Build history of the part. All positions in model axes, mm. Face numbers are marked on the shaded views. A direction names the side the tool comes from. Give positions to 0.01 mm unless a question says otherwise; leave off trailing zeros. Loops run counter-clockwise (first coordinate to the right, second up) from the corner with the lowest first, then second, coordinate; pieces in that order, holes last. Notation, with made-up numbers: (-16.75, 66.25) -> (13.25, 66.25) arc R11 ccw to (13.25, 70.25) -> close; hole circle Ø8 at (-10, 66). An arc over 180 degrees is marked (long way). Answer as a JSON object with one key per item and string values. Group by question number.
Q1. Two-plate mould, pull along X, no slides. Class the marked faces 3, 4, 5 and 6: pulls with the +X half, pulls with the -X half, needs draft (parallel to the pull), parting line crosses it, or undercut.
Q2. Wall check: probe 1 along Y at (x, z) = (-20, 0.5); probe 2 along Y at (x, z) = (21.5, 0.85). Give the ranges that are in metal, low to high. Write a range as from..to.
Q3. Tool access for the marked faces 1 and 2: list every direction of +Z, -Z, +X, -X, +Y, -Y with a clear straight run to the whole face (end or side of a thin tool).
Q4. Band-saw the part on B-B, the plane x = 26. Write the cut outline in (y, z), plus the area to 3 significant figures.
Q5. Band-saw the part on A-A, the plane y = 1.4. Count the separate pieces of the cut face and the enclosed holes in it, plus the area to 3 significant figures.
from build123d import *

# Parameters (mm, degrees)
SKETCH1_W            = 67.243323526
SKETCH1_H            = 6
BOSS_EXTRUDE1_DEPTH  = 3
CUT_EXTRUDE1_DEPTH   = 34.888289123
LPATTERN1_COUNT      = 4
LPATTERN1_PITCH      = 8
LPATTERN1_COUNT_DIR2 = 6
LPATTERN1_PITCH_DIR2 = 8


with BuildPart() as part:
    # Sketch1 → Boss-Extrude1 (new body)
    with BuildSketch(Plane.XY):
        Rectangle(SKETCH1_W, SKETCH1_H)
    extrude(amount=BOSS_EXTRUDE1_DEPTH)

    # Sketch2 → Cut-Extrude1 (cut, symmetric)
    with BuildSketch(Plane.XY):
        Polygon((0, -0.634469339), (-1.41026817, 0.075896996), (-2.589225858, 2.063475164), (-4.111542835, 3), (-4.981613855, 3.935817872), (0, 4.888597872), (4.981613855, 3.935817872), (4.111542835, 3), (2.589225858, 2.063475164), (1.41026817, 0.075896996), align=None)
    cut_extrude1 = extrude(amount=CUT_EXTRUDE1_DEPTH, both=True, mode=Mode.SUBTRACT)

    # LPattern1: Cut-Extrude1 4 × 6
    with Locations(*[Vector(-1, 0, 0) * (i * LPATTERN1_PITCH) + Vector(1, 0, 0) * (j * LPATTERN1_PITCH_DIR2) for i in range(LPATTERN1_COUNT) for j in range(LPATTERN1_COUNT_DIR2) if (i, j) != (0, 0)]):
        add(cut_extrude1, mode=Mode.SUBTRACT)


solid = part.part
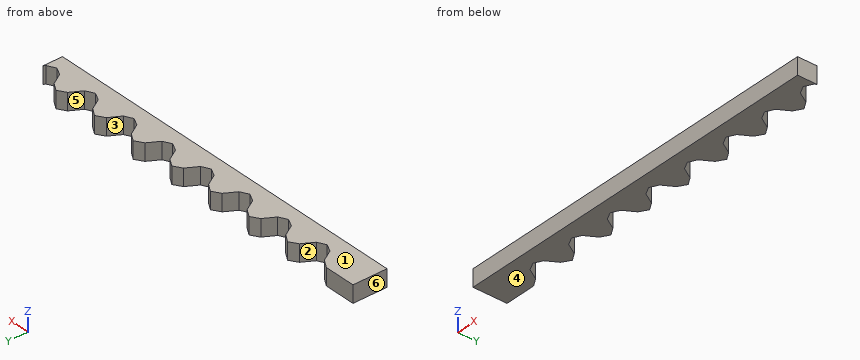
Worked answers:
{
 "1": {"face 3": "undercut", "face 4": "needs draft", "face 5": "undercut", "face 6": "pulls with the -X half"},
 "2": {"probe 1": "-3..2.93", "probe 2": "-3..1.91"},
 "3": {"face 1": "+Z, +X, -X, +Y, -Y", "face 2": "+Z, -Z, +Y"},
 "4": {"outline": "(-3, 0) -> (1.07, 0) -> (1.07, 3) -> (-3, 3) -> close", "area": "12.2 mm2"},
 "5": {"separate pieces": "8", "enclosed holes": "0", "area": "98.1 mm2"}
}
